```python
from build123d import *

# Parameters (mm, degrees)
SALIENTE_EXTRUIR2_DEPTH = 1
CROQUIS2_R              = 17.500000000000004
CROQUIS2_R_2            = 15.500000000000004
CROQUIS2_R_3            = 7.000000000000005
CROQUIS2_R_4            = 5.000000000000002
CROQUIS2_R_5            = 7.000000000010954
CROQUIS2_R_6            = 5.0000000000000036
CROQUIS2_R_7            = 7.000000000013004
CROQUIS2_R_8            = 5.000000000000005
CROQUIS2_R_9            = 6.999999999999999
CROQUIS2_R_10           = 4.999999999999999
CROQUIS2_R_11           = 7
CROQUIS2_R_12           = 4.999999999999997
CROQUIS2_R_13           = 6.999999999999995
CROQUIS2_R_14           = 5.000000000000001
SALIENTE_EXTRUIR3_DEPTH = 25
SALIENTE_EXTRUIR4_START = 1
SALIENTE_EXTRUIR4_DEPTH = 2
CROQUIS4_W              = 17.999999999999996
CROQUIS4_H              = 31.565871256335136
SALIENTE_EXTRUIR5_DEPTH = 2
CHAFL_N1_SIZE           = 2
CORTAR_EXTRUIR3_REACH   = 141.007
CROQUIS11_R             = 1.2000000000000004
CROQUIS11_R_2           = 1.200000000000001
CROQUIS11_5_R           = 1.2000000000000004
CROQUIS11_5_R_2         = 1.200000000000001
CORTAR_EXTRUIR6_DEPTH   = 9.75
MATRIZC5_COUNT          = 3
CHAFL_N4_SIZE           = 2


with BuildPart() as part:
    # Croquis1 → Saliente-Extruir2 (new body)
    with BuildSketch(Plane(origin=(0, 0, 0), x_dir=(1, 0, 0), z_dir=(0, 1, 0))):
        Polygon((-24.75, 0), (-24.75, 97), (-6.750000000000003, 97), (-6.750000000000004, 21.434128743664857), (12.375000000000004, 21.43412874366486), (96.3794641670906, -27.065871256335015), (87.3794641670906, -42.65432852445492), (21.937499999999993, -4.871392896287427), (12.375000000000004, -21.43412874366486), (-71.62946416709052, -69.93412874366491), (-80.62946416709053, -54.345671475545046), (-15.187499999999979, -16.562735847377407), align=None)
    extrude(amount=SALIENTE_EXTRUIR2_DEPTH)

    # Croquis2 → Saliente-Extruir3 (add)
    # profile 1 of 7: a face of its own
    with BuildSketch(Plane(origin=(0, 0, 0), x_dir=(1, 0, 0), z_dir=(0, 1, 0))):
        with Locations(Location((0, 0, 0), (0, 0, 270))):
            Circle(CROQUIS2_R)
        with Locations(Location((0, 0, 0), (0, 0, 270))):
            Circle(CROQUIS2_R_2, mode=Mode.SUBTRACT)
    # profile 2 of 7: a face of its own
    with BuildSketch(Plane(origin=(0, 0, 0), x_dir=(1, 0, 0), z_dir=(0, 1, 0))):
        with Locations(Location((-15.75, 88.00000000000001, 0), (0, 0, 270))):
            Circle(CROQUIS2_R_3)
        with Locations(Location((-15.75, 88.00000000000001, 0), (0, 0, 270))):
            Circle(CROQUIS2_R_4, mode=Mode.SUBTRACT)
    # profile 3 of 7: a face of its own
    with BuildSketch(Plane(origin=(0, 0, 0), x_dir=(1, 0, 0), z_dir=(0, 1, 0))):
        with Locations(Location((84.08523553304072, -30.36009989038661, 0), (0, 0, 270))):
            Circle(CROQUIS2_R_5)
        with Locations(Location((84.08523553304073, -30.360099890386614, 0), (0, 0, 270))):
            Circle(CROQUIS2_R_6, mode=Mode.SUBTRACT)
    # profile 4 of 7: a face of its own
    with BuildSketch(Plane(origin=(0, 0, 0), x_dir=(1, 0, 0), z_dir=(0, 1, 0))):
        with Locations(Location((-68.3352355330182, -57.639900109609464, 0), (0, 0, 270))):
            Circle(CROQUIS2_R_7)
        with Locations(Location((-68.3352355330182, -57.639900109609464, 0), (0, 0, 270))):
            Circle(CROQUIS2_R_8, mode=Mode.SUBTRACT)
    # profile 5 of 7: a face of its own
    with BuildSketch(Plane(origin=(0, 0, 0), x_dir=(1, 0, 0), z_dir=(0, 1, 0))):
        with Locations(Location((-15.749999999999986, 37.217064371832436, 0), (0, 0, 270))):
            Circle(CROQUIS2_R_9)
        with Locations(Location((-15.749999999999986, 37.217064371832436, 0), (0, 0, 270))):
            Circle(CROQUIS2_R_10, mode=Mode.SUBTRACT)
    # profile 6 of 7: a face of its own
    with BuildSketch(Plane(origin=(0, 0, 0), x_dir=(1, 0, 0), z_dir=(0, 1, 0))):
        with Locations(Location((40.105923200287606, -4.968632076311503, 0), (0, 0, 270))):
            Circle(CROQUIS2_R_11)
        with Locations(Location((40.105923200287606, -4.968632076311503, 0), (0, 0, 270))):
            Circle(CROQUIS2_R_12, mode=Mode.SUBTRACT)
    # profile 7 of 7: a face of its own
    with BuildSketch(Plane(origin=(0, 0, 0), x_dir=(1, 0, 0), z_dir=(0, 1, 0))):
        with Locations(Location((-24.35592320028792, -32.24843229552088, 0), (0, 0, 270))):
            Circle(CROQUIS2_R_13)
        with Locations(Location((-24.35592320028792, -32.24843229552088, 0), (0, 0, 270))):
            Circle(CROQUIS2_R_14, mode=Mode.SUBTRACT)
    extrude(amount=-SALIENTE_EXTRUIR3_DEPTH)

    # Croquis3 → Saliente-Extruir4 (add)
    with BuildSketch(Plane(origin=(0, 0, 0), x_dir=(1, 0, 0), z_dir=(0, 1, 0)).offset(SALIENTE_EXTRUIR4_START)):
        Polygon((-24.75, 97), (-6.7500000000000036, 97), (-6.7500000000000036, 53.00000000000001), (-24.749999999999993, 53.00000000000001), align=None)
        Polygon((96.37946416709256, -27.065871256333594), (58.27434640057726, -5.06587125633361), (49.27434640057727, -20.654328524453497), (87.37946416709256, -42.65432852445349), align=None)
        Polygon((-71.62946416708819, -69.93412874366587), (-33.5243464005729, -47.934128743665845), (-42.52434640057291, -32.34567147554596), (-80.6294641670882, -54.34567147554598), align=None)
        Polygon((-6.750000000000004, 21.434128743664857), (-24.75, 21.434128743664868), (-24.75, 0), (-15.187499999999979, -16.562735847377407), (-6.187499999999971, -32.151193115497286), (12.375000000000004, -21.43412874366486), (21.937499999999993, -4.871392896287427), (30.937500000000007, 10.717064371832583), (12.375000000000004, 21.43412874366486), align=None)
    extrude(amount=SALIENTE_EXTRUIR4_DEPTH)

    # Croquis4 → Saliente-Extruir5 (add)
    with BuildSketch(Plane(origin=(0, 0, 0), x_dir=(1, 0, 0), z_dir=(0, 1, 0))):
        Polygon((58.27434640057523, -5.065871256335415), (30.937500000000057, 10.717064371832285), (21.937499999999986, -4.87139289628757), (49.27434640057516, -20.654328524455266), align=None)
        with Locations((-15.750000000000002, 37.21706437183242)):
            Rectangle(CROQUIS4_W, CROQUIS4_H)
        Polygon((-33.52434640057567, -47.93412874366454), (-6.187500000000291, -32.15119311549722), (-15.187500000000146, -16.562735847377255), (-42.52434640057553, -32.34567147554457), align=None)
    extrude(amount=-SALIENTE_EXTRUIR5_DEPTH)

    # Chaflán1
    chafl_n1_edges = [part.edges().sort_by_distance(p)[0] for p in [
        (-38.02434640057291, 1, 40.139900109605904),
        (53.774346400577265, 1, 12.860099890393553),
        (-15.749999999999998, 1, -53.00000000000001),
        (-10.687499999999973, 1, 24.35696448143735),
        (26.4375, 1, -2.92283573777258),
        (-15.75, 1, -21.434128743664868),
        (-15.750000000000004, 0, -21.434128743664857),
        (-15.750000000000002, 0, -52.99999999999999),
        (26.43750000000002, 0, -2.922835737772358),
        (53.7743464005752, 0, 12.86009989039534),
        (-10.687500000000218, 0, 24.356964481437238),
        (-38.0243464005756, 0, 40.139900109604554),
    ]]
    chamfer(chafl_n1_edges, length=CHAFL_N1_SIZE - 0.0001)  # a hair under: the kernel refuses the full size

    # Croquis11 → Cortar-Extruir3 (cut, up to next)
    with BuildSketch(Plane(origin=(0, 0, 0), x_dir=(0, 0, -1), z_dir=(1, 0, 0)), mode=Mode.PRIVATE) as cortar_extruir3_sk1:
        with Locations((61.000000000000014, 1.4999999999999953)):
            Circle(CROQUIS11_R)
    cortar_extruir3_tool1 = extrude(cortar_extruir3_sk1.sketch, amount=-CORTAR_EXTRUIR3_REACH, mode=Mode.PRIVATE) & part.part
    # Croquis11 → Cortar-Extruir3 (cut, up to next)
    with BuildSketch(Plane(origin=(0, 0, 0), x_dir=(0, 0, -1), z_dir=(1, 0, 0)), mode=Mode.PRIVATE) as cortar_extruir3_sk2:
        with Locations((73.00000000000001, 1.4999999999999967)):
            Circle(CROQUIS11_R_2)
    cortar_extruir3_tool2 = extrude(cortar_extruir3_sk2.sketch, amount=-CORTAR_EXTRUIR3_REACH, mode=Mode.PRIVATE) & part.part
    # Croquis11 → Cortar-Extruir3 (cut, up to next)
    with BuildSketch(Plane(origin=(0, 0, 0), x_dir=(0, 0, -1), z_dir=(1, 0, 0)), mode=Mode.PRIVATE) as cortar_extruir3_sk3:
        with Locations((85, 1.4999999999999982)):
            Circle(CROQUIS11_R_2)
    cortar_extruir3_tool3 = extrude(cortar_extruir3_sk3.sketch, amount=-CORTAR_EXTRUIR3_REACH, mode=Mode.PRIVATE) & part.part
    cortar_extruir3_1 = cortar_extruir3_tool1.solids().sort_by_distance((0, 1.5, -61))[0]
    add(cortar_extruir3_1, mode=Mode.SUBTRACT)
    cortar_extruir3_2 = cortar_extruir3_tool2.solids().sort_by_distance((0, 1.5, -73))[0]
    add(cortar_extruir3_2, mode=Mode.SUBTRACT)
    cortar_extruir3_3 = cortar_extruir3_tool3.solids().sort_by_distance((0, 1.5, -85))[0]
    add(cortar_extruir3_3, mode=Mode.SUBTRACT)
    cortar_extruir3 = cortar_extruir3_1 + cortar_extruir3_2 + cortar_extruir3_3  # Cortar-Extruir3 as one shape, for the pattern or mirror that repeats it

    # Croquis11<5> → Cortar-Extruir6 (cut)
    with BuildSketch(Plane(origin=(0, 0, 0), x_dir=(0, 0, -1), z_dir=(1, 0, 0))):
        Polygon((54.99999999999999, -3.8e-16), (91.00000000000003, -3.8e-16), (91.00000000000009, 3), (55.00000000000002, 2.9999999999999893), align=None)
        with Locations((61.000000000000014, 1.4999999999999953)):
            Circle(CROQUIS11_5_R, mode=Mode.SUBTRACT)
        with Locations((73.00000000000001, 1.4999999999999967)):
            Circle(CROQUIS11_5_R_2, mode=Mode.SUBTRACT)
        with Locations((85, 1.4999999999999982)):
            Circle(CROQUIS11_5_R_2, mode=Mode.SUBTRACT)
    cortar_extruir6 = extrude(amount=-CORTAR_EXTRUIR6_DEPTH, mode=Mode.SUBTRACT)

    # MatrizC5: Cortar-Extruir3, Cortar-Extruir6 ×3 about axis
    matrizc5_axis = Axis((-4.81e-15, 0, 2.27e-15), (0, 1, 0))
    add([cortar_extruir3.rotate(matrizc5_axis, i * 360 / MATRIZC5_COUNT) for i in range(1, MATRIZC5_COUNT)], mode=Mode.SUBTRACT)
    add([cortar_extruir6.rotate(matrizc5_axis, i * 360 / MATRIZC5_COUNT) for i in range(1, MATRIZC5_COUNT)], mode=Mode.SUBTRACT)

    # Chaflán4
    chafl_n4_edges = [part.edges().sort_by_distance(p)[0] for p in [
        (-6.7500000000000036, 1.4999999999999996, -91.00000000000006),
        (-6.7500000000000036, 1.4999999999999944, -55.00000000000001),
        (-75.43331174438393, 1.4999999999999996, 51.34567147554506),
        (-44.25639720814411, 1.4999999999999944, 33.34567147554502),
        (82.18331174438404, 1.4999999999999996, 39.65432852445497),
        (51.00639720814418, 1.4999999999999944, 21.654328524454982),
    ]]
    chamfer(chafl_n4_edges, length=CHAFL_N4_SIZE)


solid = part.part
```
Can you work these out from the model? Positions are in its coordinate system, mm. A direction names the side the tool comes from. Round coordinates to 2 decimals unless told otherwise and drop trailing zeros. Order: outer loops, then holes, each group sorted by start corner. A loop starts at its lowest first (then second) coordinate and runs counter-clockwise, first axis right, second up. Notation, with made-up numbers: (-31, -3.5) -> (17, -3.5) arc R7 cw to (17, 4.5) -> close; hole circle Ø10 at (89.25, 35.5). An arc over 180 degrees is marked (long way). Return JSON: item names as keys, results as strings. Group by question number.
1. If we section it at B-B, the plane x = 0: Write out the boundary of the cut face in (y, z).
2. If we section it at A-A, the plane y = -22: Count the separate pieces of the cut face and the enclosed holes in it, then the cut area to 3 significant figures.
3. I need wall thicknesses on line 1 (X direction, y = -20.5, z = 28); line 2 (Z direction, x = -1, y = -10.5); line 3 (Z direction, x = -19, y = -5.5). Which ranges of each line are inside material? Lowest first, please. Write a range as [from, to].
4. We'd pull the mould along Z, two halves only. Please class faces 1 (the face through (54.589, -0.986, 13.476)), 2 (the face through (-55.61, 1.04, 51.9)), 3 (the face through (-20, -25, -34)): released by +Z, released by -Z, zero draft, split by the parting line, or undercut.
5. If we section it at C-C, the plane x = 43: Write out the boundary of the cut face in (y, z).
6. Which directions (+Z, -Z, +X, -X, +Y, -Y) give clear straight access to the entire face, cutting with the end or side of a thin tool? Please do faces 4 (the face through (71, 0, 22)), 5 (the face through (-24.75, 0, -48)), 6 (the face through (17.66, 1.48, 12.28)).
7. Will these pins go through, and if not, where does the flat tip stop? pin 1 (2 mm diameter, centred on y = -15.5, z = -7, fed in from -X); pin 2 (4 mm diameter, centred on y = -3, z = -77, fed in from -X); pin 3 (15.5 mm diameter, centred on x = 40, z = 7, fed in from -Y); pin 4 (3 mm diameter, centred on y = 1.5, z = -85, fed in from -X).
Output values:
{
 "1": {"outline": "(-25, -17.5) -> (0, -17.5) -> (0, -21.43) -> (3, -21.43) -> (3, 28.58) -> (0, 28.58) -> (0, 17.5) -> (-25, 17.5) -> (-25, 15.5) -> (0, 15.5) -> (0, -15.5) -> (-25, -15.5) -> close"},
 "2": {"separate pieces": "7", "enclosed holes": "7", "area": "660 mm²"},
 "3": {"line 1": "[-29.92, -26.99], [-21.72, -18.79], [77.5, 79.68], [88.49, 90.68]", "line 2": "[-17.47, -15.47], [15.47, 17.47]", "line 3": "[-94.2, -91.8], [-84.2, -81.8], [-43.42, -41.02], [-33.42, -31.02], [27.74, 36.76]"},
 "4": {"face 1": "released by +Z", "face 2": "undercut", "face 3": "zero draft"},
 "5": {"outline": "(-25, -1.41) -> (-2, -1.41) -> (-2, -3.75) -> (1, -3.75) -> (1, 17.03) -> (-2, 17.03) -> (-2, 11.34) -> (-25, 11.34) -> (-25, 9.05) -> (-2, 9.05) -> (-2, 0.89) -> (-25, 0.89) -> close"},
 "6": {"face 4": "-Y", "face 5": "-Z, -X, +Y, -Y", "face 6": "+Z, +Y, -Y"},
 "7": {"pin 1": "x = -16.44", "pin 2": "through", "pin 3": "y = -25", "pin 4": "x = -24.75"}
}
